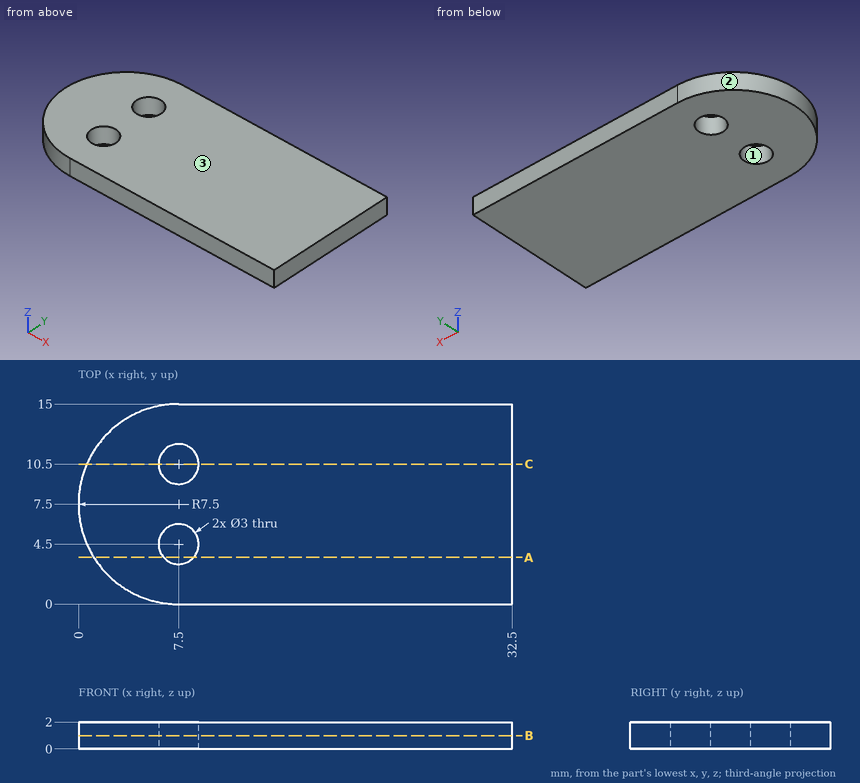
For this review, use the dimensioned drawing (mm, ordinates from the lowest corner) and the shaded views. Give positions to 0.01 mm unless a question says otherwise; leave off trailing zeros. Write each loop counter-clockwise with the first axis right and the second up, starting at its lowest first coordinate (ties: lowest second). Pieces come first, ordered by that corner, then holes. Notation, with made-up numbers: M 56.25,81 L 85.25,81 A17 cw 85.25,108 Z; hole C 15.5,12 d5. An arc over 180 degrees is marked long. Write item = value, one per line. Start each with the question number.
Q1. We need section A-A (y = 3.5). State the section outline as (x, z) points.
Q2. We need section C-C (y = 10.5). State the section outline as (x, z) points.
Q3. For line 1 (Y direction, x = 7.5, z = 0.3); line 2 (X direction, y = 5.25, z = 0.3); line 3 (X direction, y = 12.75, z = 1.8), list the stretches that pass through material, from the lowest coordinate up.
Q4. Mouldability with a two-part tool opening along X and no side actions: class the marked faces 1, 2 and 3 as released by +X, released by -X, zero draft, split by the parting line, or undercut.
Q5. We need section B-B (z = 1). State the section outline as (x, y) points, plus the area to 3 significant figures.
Result set:
q1.outline = M 1.16,0 L 6.38,0 L 6.38,2 L 1.16,2 Z; M 8.62,0 L 32.5,0 L 32.5,2 L 8.62,2 Z
q2.outline = M 0.63,0 L 6,0 L 6,2 L 0.63,2 Z; M 9,0 L 32.5,0 L 32.5,2 L 9,2 Z
q3.line_1 = 0 to 3, 6 to 9, 12 to 15
q3.line_2 = 0.35 to 6.2, 8.8 to 32.5
q3.line_3 = 2.14 to 32.5
q4.face_1 = undercut
q4.face_2 = released by -X
q4.face_3 = zero draft
q5.outline = M 7.5,0 L 32.5,0 L 32.5,15 L 7.5,15 A7.5 ccw Z; hole C 7.5,4.5 d3; hole C 7.5,10.5 d3
q5.area = 449 mm2
